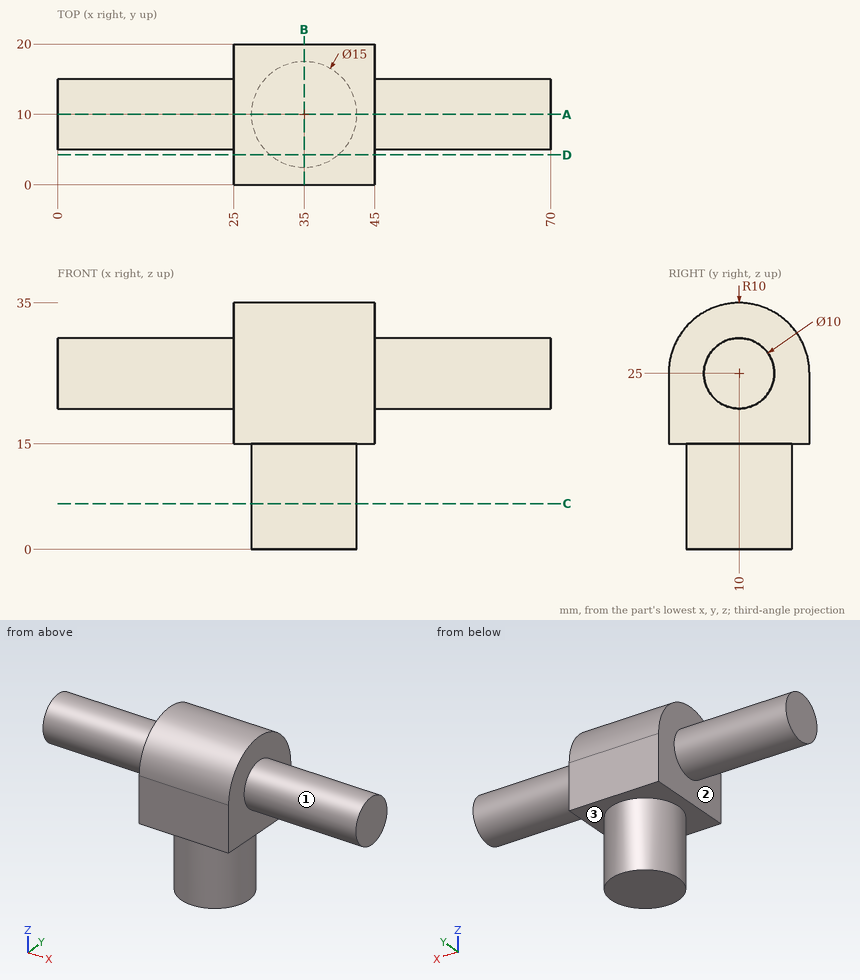
Drawing for the job (mm, zero at the part's lowest x, y, z). A direction names the side the tool comes from. Round coordinates to 2 decimals unless told otherwise and drop trailing zeros. Loops run counter-clockwise (first coordinate to the right, second up) from the corner with the lowest first, then second, coordinate; pieces in that order, holes last. Notation, with made-up numbers: (19.5, -19) - (26.5, -19) arc R29 ccw to (26.5, 8) - close; hole circle Ø5 at (2, -29.75). An arc over 180 degrees is marked (long way). Return JSON: item names as keys, results as strings. Group by question number.
Q1. Band-saw the part on B-B on x = 35. Give the cut face in (y, z), plus the area to 3 significant figures.
Q2. Band-saw the part on A-A on y = 10. Give the cut face in (x, z), plus the area to 4 significant figures.
Q3. Tool access for the marked faces 1, 2 and 3: list every direction of +Z, -Z, +X, -X, +Y, -Y with a clear straight run to the whole face (end or side of a thin tool).
Q4. Flat gauge pins, fed straight in: pin 1 Ø3 at (y, z) = (11.5, 4.5) entering from -X; pin 2 Ø3 at (y, z) = (12.5, 11.5) entering from -X; pin 3 Ø1 at (x, y) = (47, 7.5) entering from +Z. Where does each tip first touch, or does it go through?
Q5. Band-saw the part on C-C on z = 6.5. Give the cut face in (x, y).
Q6. Band-saw the part on D-D on y = 4.25. Give the cut face in (x, z).
Q7. Drill centre lines: line 1 along X through (y, z) = (10.5, 17); line 2 along Y through (x, z) = (65.5, 23.5); line 3 along Z through (x, y) = (36, 5.75). Where is each one in solid material? Low to high. Write a range as [from, to].
Solutions:
{
 "1": {"outline": "(0, 15) - (2.5, 15) - (2.5, 0) - (17.5, 0) - (17.5, 15) - (20, 15) - (20, 25) arc R10 ccw to (0, 25) - close", "area": "582 mm^2"},
 "2": {"outline": "(0, 20) - (25, 20) - (25, 15) - (27.5, 15) - (27.5, 0) - (42.5, 0) - (42.5, 15) - (45, 15) - (45, 20) - (70, 20) - (70, 30) - (45, 30) - (45, 35) - (25, 35) - (25, 30) - (0, 30) - close", "area": "1,125 mm^2"},
 "3": {"face 1": "+X", "face 2": "-X", "face 3": "-Z"},
 "4": {"pin 1": "stops at x = 27.5", "pin 2": "stops at x = 27.57", "pin 3": "stops at z = 29.58"},
 "5": {"outline": "circle Ø15 at (35, 10)"},
 "6": {"outline": "(25, 15) - (30.18, 15) - (30.18, 0) - (39.82, 0) - (39.82, 15) - (45, 15) - (45, 33.18) - (25, 33.18) - close"},
 "7": {"line 1": "x = [25, 45]", "line 2": "y = [5.23, 14.77]", "line 3": "z = [0, 34.05]"}
}
